Autodesk Inventor part; units mm, degrees
ref_plane "YZ Plane" through (0, 0, 0) normal (1, 0, 0) x (0, 1, 0)
ref_plane "XZ Plane" through (0, 0, 0) normal (0, 1, 0) x (-1, 0, 0)
ref_plane "XY Plane" through (0, 0, 0) normal (0, 0, 1) x (1, 0, 0)
sketch "Sketch1" plane through (0, 0, 0) normal (0, 0, 1) x (1, 0, 0)
  line L0 (0, 0) -> (15, 0)
  line L1 (15, 0) -> (15, 15)
  line L2 (15, 15) -> (0, 15)
  line L3 (0, 15) -> (0, 0)
  dimension "d0" = 15
  dimension "d1" = 15
extrude "Extrusion1" add sketch "Sketch1" along normal blind 10
sketch "Sketch2" plane through (0, 0, 10) normal (0, 0, 1) x (1, 0, 0)
  line L0 (0, 15) -> (7.1003, 15)
  line L1 (15, 15) -> (0, 15)
  line L2 (7.5, 15) -> (7.5, 0)
  line L3 (0, 15) -> (7.9375, 15)
  line L4 (0, 0) -> (0, 7.9375)
  line L5 (0, 7.9375) -> (15, 7.9375)
  circle A0 centre (7.5, 7.9375) radius 4.5
  dimension "d15" = 9
extrude "Extrusion2" add sketch "Sketch2" along normal blind 250
thread "Thread1"
ref_plane "Work Plane1" through (7.5, 7.9375, 260) normal (0, 0, 1) x (1, 0, 0)
sketch "Sketch3" plane through (7.5, 7.9375, 260) normal (0, 0, 1) x (1, 0, 0)
  circle A0 centre (0, 0) radius 5.5
  circle A1 centre (0, 0) radius 4.5
  point P0 (-7.5, -7.9375)
  dimension "d10" = 9
extrude "Extrusion3" add sketch "Sketch3" along normal blind 50 contours A1
thread "Thread2"
properties part number "nut1"
Geometry check sheet. Reference: the model listing, model coordinates, mm. A direction names the side the tool comes from. Round coordinates to 2 decimals unless told otherwise and drop trailing zeros. Order: outer loops, then holes, each group sorted by start corner. A loop starts at its lowest first (then second) coordinate and runs counter-clockwise, first axis right, second up. Notation, with made-up numbers: M 28.25,-37 L 52.25,-37 A24 cw 52.25,-19 Z; hole C 17,36.5 d7. An arc over 180 degrees is marked long. Write item = value, one per line.
Q1. Section check A-A (x = 7.5). Enter the section's corners in (y, z), plus the area to 3 significant figures.
Answer block:
outline = M 0,0 L 15,0 L 15,10 L 12.44,10 L 12.44,310 L 3.44,310 L 3.44,10 L 0,10 Z
area = 2,850 mm^2
Q2. Set-up check for faces 1 (the cylindrical face through (11.657, 9.661, 157.9)), 2 (the flat face through (8, 15, 5)): record each of +Z, -Z, +X, -X, +Y, -Y from which the full face is reachable in a straight line by a thin tool's end or side.
Answer block:
face_1 = +Z
face_2 = +Z, -Z, +X, -X, +Y
Q3. Scan lines: line 1 (Z direction, x = 0.5, y = 0.5); line 2 (X direction, y = 7.25, z = 82); line 3 (Y direction, x = 7.5, z = 194). Record each from-to range of solid material in increasing order.
Answer block:
line_1 = 0 to 10
line_2 = 3.05 to 11.95
line_3 = 3.44 to 12.44
Q4. Depth check by flat-ended pin: pin 1 Ø5 at (y, z) = (12, 170.5) entering from -X; pin 2 Ø6 at (x, z) = (4.5, 103) entering from +Y; pin 3 Ø2 at (y, z) = (7.5, 72.5) entering from -X. Enter the tip coordinate at first touch or a pass-through.
Answer block:
pin_1 = 3.28
pin_2 = 12.44
pin_3 = 3
Q5. Section check B-B (z = 147). Enter the section's corners in (x, y), plus the area to 3 significant figures.
Answer block:
outline = C 7.5,7.94 d9
area = 63.6 mm^2
